Geometry: final body of the model. Coordinates: model frame, mm. A direction names the side the tool comes from. Give positions to 0.01 mm unless a question says otherwise; leave off trailing zeros. Write each loop counter-clockwise with the first axis right and the second up, starting at its lowest first coordinate (ties: lowest second). Pieces come first, ordered by that corner, then holes.
Q1. Draft query along Y for faces 1 (the face through (-4, 1, 12.7)), 2 (the face through (258.78, -45.96, 12.07)), 3 (the face through (259.2, 43.57, 12.07)). Return one class per face: pulls with the +Y half, pulls with the -Y half, needs draft (parallel to the pull), parting line crosses it, or undercut.
Q2. Line query: L1, parallel to Y at x = 1.5, z = 5.5 (3 decimals); L2, parallel to Z at x = 225.5, y = -54.5; L3, parallel to Y at x = 191.5, z = 1. Output: solid intervals per line, ascending.
Q3. Reachability of faces 4 (the face through (4, 1, 11.43)), 5 (the face through (-320.675, 0, 12)) from +Z, -Z, +X, -X, +Y, -Y: full face, straight path, thin tool, end or side. Return the list, or none.
Q4. Pin query (flat end, axial travel): pin 1 (1 mm diameter, centred on x = -121.5, y = 67.5, fed in from -Z); pin 2 (9 mm diameter, centred on x = -66.68, y = 90.49, fed in from +Z); pin 3 (6.5 mm diameter, centred on x = 253.619, y = -43.815, fed in from -Z); pin 4 (2 mm diameter, centred on x = 255.5, z = 11.5, fed in from +Y). Return the tip coordinate at first contact, or that it passes through.
Q5. Cut plane A-A on x = -216.5. Return the cut outline in (y, z) (3 decimals).
Q6. Cut plane B-B on y = -24. Return the cut outline in (x, z) (3 decimals).
```python
from build123d import *

# Parameters (mm, degrees)
SKETCH1_W           = 641.35
SKETCH1_H           = 190.5
BOSS_EXTRUDE1_DEPTH = 12.7
SKETCH2_W           = 641.35
SKETCH2_H           = 12.7
CUT_EXTRUDE1_DEPTH  = 11.43
SKETCH4_W           = 641.35
SKETCH4_H           = 158.75
CUT_EXTRUDE2_DEPTH  = 11.43
FILLET2_R           = 3.175
SKETCH6_R           = 3.429
CUT_EXTRUDE3_DEPTH  = 11.43
SKETCH8_R           = 5.588
CUT_EXTRUDE4_DEPTH  = 11.43
SKETCH9_R           = 3.429
CUT_EXTRUDE5_DEPTH  = 11.43


with BuildPart() as part:
    # Sketch1 → Boss-Extrude1 (new body)
    with BuildSketch(Plane.XY):
        Rectangle(SKETCH1_W, SKETCH1_H)
    extrude(amount=BOSS_EXTRUDE1_DEPTH)

    # Sketch2 → Cut-Extrude1 (cut)
    with BuildSketch(Plane.XY.offset(12.7)):
        with Locations((0, 88.9)):
            Rectangle(SKETCH2_W, SKETCH2_H)
        with Locations((0, -88.9)):
            Rectangle(SKETCH2_W, SKETCH2_H)
    extrude(amount=-CUT_EXTRUDE1_DEPTH, mode=Mode.SUBTRACT)

    # Sketch4 → Cut-Extrude2 (cut)
    with BuildSketch(Plane(origin=(0, 0, 0), x_dir=(-1, 0, 0), z_dir=(0, 0, -1))):
        Rectangle(SKETCH4_W, SKETCH4_H)
    extrude(amount=-CUT_EXTRUDE2_DEPTH, mode=Mode.SUBTRACT)

    # Fillet2
    fillet2_edges = [part.edges().sort_by_distance(p)[0] for p in [
        (0, 82.55, 1.27),
        (0, 82.55, 12.7),
        (0, -82.55, 12.7),
        (0, -82.55, 1.27),
        (0, 79.375, 0),
        (0, -79.375, 11.43),
        (0, 79.375, 11.43),
        (0, -79.375, 0),
    ]]
    fillet(fillet2_edges, radius=FILLET2_R)

    # Sketch6 → Cut-Extrude3 (cut)
    with BuildSketch(Plane.XY.offset(1.27)):
        with Locations((-286.385, 90.4875)):
            Circle(SKETCH6_R)
        with Locations((-242.443, 90.4875)):
            Circle(SKETCH6_R)
        with Locations((-198.501, 90.4875)):
            Circle(SKETCH6_R)
        with Locations((-154.559, 90.4875)):
            Circle(SKETCH6_R)
        with Locations((-110.617, 90.4875)):
            Circle(SKETCH6_R)
        with Locations((-66.675, 90.4875)):
            Circle(SKETCH6_R)
        with Locations((-22.733, 90.4875)):
            Circle(SKETCH6_R)
        with Locations((21.209, 90.4875)):
            Circle(SKETCH6_R)
        with Locations((65.151, 90.4875)):
            Circle(SKETCH6_R)
        with Locations((109.093, 90.4875)):
            Circle(SKETCH6_R)
        with Locations((153.035, 90.4875)):
            Circle(SKETCH6_R)
        with Locations((196.977, 90.4875)):
            Circle(SKETCH6_R)
        with Locations((240.919, 90.4875)):
            Circle(SKETCH6_R)
        with Locations((284.861, 90.4875)):
            Circle(SKETCH6_R)
        with Locations(Location((284.861, -90.4875, 0), (0, 0, 180))):
            Circle(SKETCH6_R)
        with Locations(Location((240.919, -90.4875, 0), (0, 0, 180))):
            Circle(SKETCH6_R)
        with Locations(Location((196.977, -90.4875, 0), (0, 0, 180))):
            Circle(SKETCH6_R)
        with Locations(Location((153.035, -90.4875, 0), (0, 0, 180))):
            Circle(SKETCH6_R)
        with Locations(Location((109.093, -90.4875, 0), (0, 0, 180))):
            Circle(SKETCH6_R)
        with Locations(Location((65.151, -90.4875, 0), (0, 0, 180))):
            Circle(SKETCH6_R)
        with Locations(Location((21.209, -90.4875, 0), (0, 0, 180))):
            Circle(SKETCH6_R)
        with Locations(Location((-22.733, -90.4875, 0), (0, 0, 180))):
            Circle(SKETCH6_R)
        with Locations(Location((-66.675, -90.4875, 0), (0, 0, 180))):
            Circle(SKETCH6_R)
        with Locations(Location((-110.617, -90.4875, 0), (0, 0, 180))):
            Circle(SKETCH6_R)
        with Locations(Location((-154.559, -90.4875, 0), (0, 0, 180))):
            Circle(SKETCH6_R)
        with Locations(Location((-198.501, -90.4875, 0), (0, 0, 180))):
            Circle(SKETCH6_R)
        with Locations(Location((-242.443, -90.4875, 0), (0, 0, 180))):
            Circle(SKETCH6_R)
        with Locations(Location((-286.385, -90.4875, 0), (0, 0, 180))):
            Circle(SKETCH6_R)
    extrude(amount=-CUT_EXTRUDE3_DEPTH, mode=Mode.SUBTRACT)

    # Sketch8 → Cut-Extrude4 (cut)
    with BuildSketch(Plane.XY.offset(12.7)):
        with Locations((-253.619, 43.815)):
            Circle(SKETCH8_R)
        with Locations(Location((253.619, 43.815, 0), (0, 0, 180))):
            Circle(SKETCH8_R)
        with Locations((253.619, -43.815)):
            Circle(SKETCH8_R)
        with Locations(Location((-253.619, -43.815, 0), (0, 0, 180))):
            Circle(SKETCH8_R)
    extrude(amount=-CUT_EXTRUDE4_DEPTH, mode=Mode.SUBTRACT)

    # Sketch9 → Cut-Extrude5 (cut)
    with BuildSketch(Plane.XY.offset(12.7)):
        with Locations((-206.375, 44.015279051)):
            Circle(SKETCH9_R)
        with Locations(Location((206.375, 44.015279051, 0), (0, 0, 180))):
            Circle(SKETCH9_R)
        with Locations((206.375, -44.015279051)):
            Circle(SKETCH9_R)
        with Locations(Location((-206.375, -44.015279051, 0), (0, 0, 180))):
            Circle(SKETCH9_R)
    extrude(amount=-CUT_EXTRUDE5_DEPTH, mode=Mode.SUBTRACT)


solid = part.part
```
Data:
1. face 1: needs draft
1. face 2: undercut
1. face 3: undercut
2. L1: y = -82.55 to -79.375, 79.375 to 82.55
2. L2: z = 11.43 to 12.7
2. L3: y = -95.25 to -80.24, 80.24 to 95.25
3. face 4: -Z, +X, -X
3. face 5: +Z, -Z, -X, +Y, -Y
4. pin 1: stops at z = 11.43
4. pin 2: stops at z = 1.27
4. pin 3: passes through
4. pin 4: stops at y = 82.4
5. outline: (-95.25, 0) - (-82.55, 0) arc R3.175 ccw to (-79.375, 3.175) - (-79.375, 8.255) arc R3.175 cw to (-76.2, 11.43) - (76.2, 11.43) arc R3.175 cw to (79.375, 8.255) - (79.375, 3.175) arc R3.175 ccw to (82.55, 0) - (95.25, 0) - (95.25, 1.27) - (85.725, 1.27) arc R3.175 cw to (82.55, 4.445) - (82.55, 9.525) arc R3.175 ccw to (79.375, 12.7) - (-79.375, 12.7) arc R3.175 ccw to (-82.55, 9.525) - (-82.55, 4.445) arc R3.175 cw to (-85.725, 1.27) - (-95.25, 1.27) - close
6. outline: (-320.675, 11.43) - (320.675, 11.43) - (320.675, 12.7) - (-320.675, 12.7) - close
